Source: CAD feature listing. Evaluate the final solid. Frame: model axes, mm. Face numbers are marked on the shaded views. A direction names the side the tool comes from. Give positions to 0.01 mm unless a question says otherwise; leave off trailing zeros. Write each loop counter-clockwise with the first axis right and the second up, starting at its lowest first coordinate (ties: lowest second). Pieces come first, ordered by that corner, then holes. Notation, with made-up numbers: M -16,47.5 L -9,47.5 A20 ccw -9,77.5 Z; hole C 80.25,83 d9. An arc over 180 degrees is marked long. Return JSON: item names as keys, results as strings.
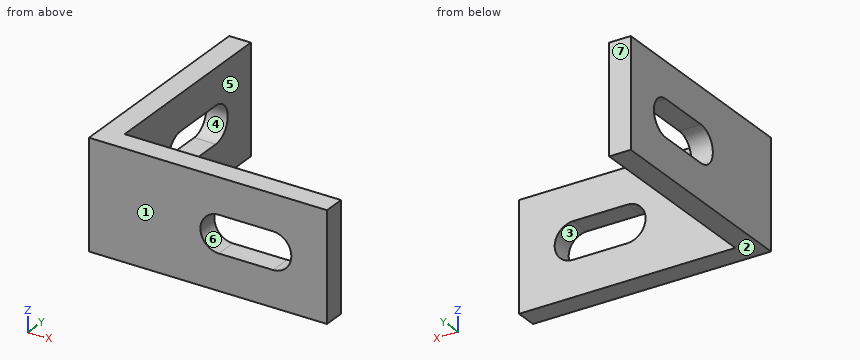
```python
from build123d import *

# Parameters (mm, degrees)
SKETCH_1_W      = 20
SKETCH_1_H      = 10
EXTRUDE_1_DEPTH = 2
SKETCH_3_W      = 10
SKETCH_3_H      = 20
EXTRUDE_3_DEPTH = 2


with BuildPart() as part:
    # 草图1 → 凸台-拉伸1 (new body)
    with BuildSketch(Plane(origin=(0, 0, 0), x_dir=(1, 0, 0), z_dir=(0, 1, 0))):
        Rectangle(SKETCH_1_W, SKETCH_1_H)
        with BuildLine():
            Line((5, -1.7), (0, -1.7))
            ThreePointArc((0, -1.7), (-1.7, 0), (0, 1.7))
            Line((0, 1.7), (5, 1.7))
            ThreePointArc((5, 1.7), (6.7, 0), (5, -1.7))
        make_face(mode=Mode.SUBTRACT)
    extrude(amount=EXTRUDE_1_DEPTH)

    # 草图3 → 凸台-拉伸3 (add)
    with BuildSketch(Plane.ZY.offset(10)):
        with Locations((0, 10)):
            Rectangle(SKETCH_3_W, SKETCH_3_H)
        with BuildLine():
            Line((1.7, 15), (1.7, 10))
            ThreePointArc((1.7, 10), (0, 8.3), (-1.7, 10))
            Line((-1.7, 10), (-1.7, 15))
            ThreePointArc((-1.7, 15), (0, 16.7), (1.7, 15))
        make_face(mode=Mode.SUBTRACT)
    extrude(amount=EXTRUDE_3_DEPTH)


solid = part.part
```
1) Contact query for flat-ended pins moving along their axis: pin 1 Ø3 at (x, z) = (-1.5, -1.5) entering from +Y; pin 2 Ø4 at (y, z) = (5.5, -1.5) entering from +X. Output: stop coordinate, or through.
Numbers:
{"pin 1": "stops at y = 2", "pin 2": "stops at x = -10"}
2) Cut plane D-D, the plane z = 2.25. Return the cut outline in (x, y), then the cut area to 3 significant figures.
Numbers:
{"outline": "M -12,0 L 10,0 L 10,2 L -10,2 L -10,20 L -12,20 Z", "area": "80.0 mm²"}
3) Draft query along Z for the marked faces 1, 2 and 3. Return one class per face: released by +Z, released by -Z, zero draft, split by the parting line, or undercut.
Numbers:
{"face 1": "zero draft", "face 2": "released by -Z", "face 3": "undercut"}
4) Line query: line 1 (Z direction, x = 3.25, y = 1); line 2 (Y direction, x = 1.25, z = -2.5); line 3 (X direction, y = 10.75, z = -4). Output: solid intervals per line, ascending. Write a range as [from, to].
Numbers:
{"line 1": "z = [-5, -1.7], [1.7, 5]", "line 2": "y = [0, 2]", "line 3": "x = [-12, -10]"}
5) Cut plane C-C, the plane x = -10.5. Return the cut outline in (y, z), then the cut area to 3 significant figures.
Numbers:
{"outline": "M 0,-5 L 20,-5 L 20,5 L 0,5 Z; hole M 10,-1.7 L 15,-1.7 A1.7 ccw 15,1.7 L 10,1.7 A1.7 ccw Z", "area": "174 mm²"}
6) Cut plane B-B, the plane y = 13.5. Return the cut outline in (x, z).
Numbers:
{"outline": "M -12,-5 L -10,-5 L -10,-1.7 L -12,-1.7 Z; M -12,1.7 L -10,1.7 L -10,5 L -12,5 Z"}
7) Set-up query: the marked faces 4, 5, 6 and 7. Return all of +Z, -Z, +X, -X, +Y, -Y with unobstructed straight access to the full face (end or side cutting, diameter ignored); none if empty.
Numbers:
{"face 4": "+X, -X", "face 5": "+Z, -Z, +X, +Y", "face 6": "+Y, -Y", "face 7": "+Z, -Z, +X, -X, +Y"}
8) Cut plane A-A, the plane x = 0.75. Return the cut outline in (y, z).
Numbers:
{"outline": "M 0,-5 L 2,-5 L 2,-1.7 L 0,-1.7 Z; M 0,1.7 L 2,1.7 L 2,5 L 0,5 Z"}
